For this review, take the finished solid that the model builds, in its own axes (mm). A direction names the side the tool comes from. Give positions to 0.01 mm unless a question says otherwise; leave off trailing zeros. Order: outer loops, then holes, each group sorted by start corner. A loop starts at its lowest first (then second) coordinate and runs counter-clockwise, first axis right, second up. Notation, with made-up numbers: (-33.5, -29) -> (0.5, -29) arc R21 cw to (0.5, -20) -> close; hole circle Ø6 at (28, 20). An arc over 180 degrees is marked (long way). Return JSON: item names as keys, results as strings. Group by question number.
1) Add section D-D (z = -24.5). Give the boundary of the cut face in (x, y).
2) The part is to be moulded in two halves that separate along Z. For faces 3 (the face through (0, 1, 29.5)), 4 (the face through (-27.89, 0.99, -23.49)), 5 (the face through (10.15, 1, 0)), 6 (the face through (-34.918, 1, 0)), say which applies: released by +Z, released by -Z, zero draft, split by the parting line, or undercut.
3) Add section C-C (x = -29.5). Give the boundary of the cut face in (y, z).
4) For faces 1 (the face through (7.9, 1, 5.5)), 2 (the face through (0, 1, -29.5)), list the 3-axis set-ups (+Z, -Z, +X, -X, +Y, -Y) from which the entire face can be reached by the end or side of a thin tool; tool diameter is ignored.
5) To check wall thickness, follow line 1 along Z through (x, y) = (0, 1.1); line 2 along Z through (x, y) = (3.5, 0.55); line 3 along X through (y, z) = (1.25, 24). State the ranges of each line that lie inside material, in increasing order.
6) Insertion check: P1, Ø1.8, axis at x = -29, z = 24.5, coming from the +Y side; P2, Ø21, axis at x = 0, z = 13.48, coming from the +Y side. Each pin has a flat end and moves straight along its axis. Give the tip position at first contact, or say it passes through.
7) Add section B-B (y = 1.65). Give the boundary of the cut face in (x, z).
8) Add section A-A (z = 4). Give the boundary of the cut face in (x, y), then the cut area to 3 significant figures.
from build123d import *

# Parameters (mm, degrees)
SKETCH_2_W      = 69.836734694
SKETCH_2_H      = 59
SKETCH_2_R      = 8
SKETCH_2_R_2    = 1.5
EXTRUDE_1_DEPTH = 2
FILLET_1_R      = 7


with BuildPart() as part:
    # 草圖2 → 填料-伸長1 (new body)
    with BuildSketch(Plane(origin=(0, 0, 0), x_dir=(-1, 0, 0), z_dir=(0, 1, 0))):
        Rectangle(SKETCH_2_W, SKETCH_2_H)
        with Locations((0, 13.48)):
            Circle(SKETCH_2_R, mode=Mode.SUBTRACT)
        with Locations((0, -13.48)):
            Circle(SKETCH_2_R, mode=Mode.SUBTRACT)
        with Locations((29, 24.5)):
            Circle(SKETCH_2_R_2, mode=Mode.SUBTRACT)
        with Locations((29, -24.5)):
            Circle(SKETCH_2_R_2, mode=Mode.SUBTRACT)
        with Locations((-29, 24.5)):
            Circle(SKETCH_2_R_2, mode=Mode.SUBTRACT)
        with Locations((-29, -24.5)):
            Circle(SKETCH_2_R_2, mode=Mode.SUBTRACT)
        with BuildLine():
            Line((-5.65, 3.25), (-5.65, -3.25))
            ThreePointArc((-5.65, -3.25), (-7.9, -5.5), (-10.15, -3.25))
            Line((-10.15, -3.25), (-10.15, 3.25))
            ThreePointArc((-10.15, 3.25), (-7.9, 5.5), (-5.65, 3.25))
        make_face(mode=Mode.SUBTRACT)
    extrude(amount=EXTRUDE_1_DEPTH)

    # 圓角1
    fillet_1_edges = [part.edges().sort_by_distance(p)[0] for p in [
        (-34.918367347, 1, -29.5),
        (34.918367347, 1, -29.5),
        (34.918367347, 1, 29.5),
        (-34.918367347, 1, 29.5),
    ]]
    fillet(fillet_1_edges, radius=FILLET_1_R)


solid = part.part
Evaluation:
{
 "1": {"outline": "(-34.63, 0) -> (-30.5, 0) -> (-30.5, 2) -> (-34.63, 2) -> close; (-27.5, 0) -> (27.5, 0) -> (27.5, 2) -> (-27.5, 2) -> close; (30.5, 0) -> (34.63, 0) -> (34.63, 2) -> (30.5, 2) -> close"},
 "2": {"face 3": "released by +Z", "face 4": "undercut", "face 5": "undercut", "face 6": "zero draft"},
 "3": {"outline": "(0, -29.32) -> (2, -29.32) -> (2, -25.91) -> (0, -25.91) -> close; (0, -23.09) -> (2, -23.09) -> (2, 23.09) -> (0, 23.09) -> close; (0, 25.91) -> (2, 25.91) -> (2, 29.32) -> (0, 29.32) -> close"},
 "4": {"face 1": "+Y, -Y", "face 2": "-Z, +X, -X, +Y, -Y"},
 "5": {"line 1": "-29.5 to -21.48, -5.48 to 5.48, 21.48 to 29.5", "line 2": "-29.5 to -20.67, -6.29 to 6.29, 20.67 to 29.5", "line 3": "-34.76 to -30.41, -27.59 to 27.59, 30.41 to 34.76"},
 "6": {"P1": "through", "P2": "y = 2"},
 "7": {"outline": "(-34.92, -22.5) arc R7 ccw to (-27.92, -29.5) -> (27.92, -29.5) arc R7 ccw to (34.92, -22.5) -> (34.92, 22.5) arc R7 ccw to (27.92, 29.5) -> (-27.92, 29.5) arc R7 ccw to (-34.92, 22.5) -> close; hole circle Ø3 at (-29, -24.5); hole circle Ø3 at (-29, 24.5); hole circle Ø16 at (0, -13.48); hole circle Ø16 at (0, 13.48); hole (5.65, -3.25) arc R2.25 ccw to (10.15, -3.25) -> (10.15, 3.25) arc R2.25 ccw to (5.65, 3.25) -> close; hole circle Ø3 at (29, -24.5); hole circle Ø3 at (29, 24.5)"},
 "8": {"outline": "(-34.92, 0) -> (5.78, 0) -> (5.78, 2) -> (-34.92, 2) -> close; (10.02, 0) -> (34.92, 0) -> (34.92, 2) -> (10.02, 2) -> close", "area": "131 mm^2"}
}
